from build123d import *

# Parameters (mm, degrees)
F0_R     = 12.942623
F1_DEPTH = 4.064
F4_DEPTH = 25.4
F5_DEPTH = 25.4


with BuildPart() as f1:
    # F0 (on Top) → F1 (new body)
    with BuildSketch(Plane.XY):
        Circle(F0_R)
    extrude(amount=F1_DEPTH)

    # F2 (on Top) → F4 (join)
    with BuildSketch(Plane.XY):
        Polygon((1.975973, 9.017531), (1.975973, 11.293087), (0.005284, 12.430865), (-1.965406, 11.293087), (-1.965406, 9.017531), (0.005284, 7.879752), align=None)
    extrude(amount=F4_DEPTH)

    # F3 (on face) → F5 (join)
    with BuildSketch(Plane.XY):
        Polygon((1.963999, -11.134515), (1.963999, -8.858958), (-0.006691, -7.72118), (-1.977381, -8.858958), (-1.977381, -11.134515), (-0.006691, -12.272293), align=None)
    extrude(amount=F5_DEPTH)


solid = f1.part
Input: part model. Units: mm. Frame: model coordinates. A direction names the side the tool comes from. Round coordinates to 2 decimals unless told otherwise and drop trailing zeros. Order: outer loops, then holes, each group sorted by start corner. A loop starts at its lowest first (then second) coordinate and runs counter-clockwise, first axis right, second up.
1. Cut plane D-D, the plane y = -9.5. Output: boundary loops of the cut face in (x, z), then the cut area to 3 significant figures.
The answers:
outline: (-8.79, 0) - (8.79, 0) - (8.79, 4.06) - (1.96, 4.06) - (1.96, 25.4) - (-1.98, 25.4) - (-1.98, 4.06) - (-8.79, 4.06) - close
area: 156 mm2
2. Cut plane B-B, the plane y = 0. Output: boundary loops of the cut face in (x, z), then the cut area to 3 significant figures.
The answers:
outline: (-12.94, 0) - (12.94, 0) - (12.94, 4.06) - (-12.94, 4.06) - close
area: 105 mm2
3. Material intervals for line 1 (Y direction, x = 0, z = 14.25); line 2 (Z direction, x = -6, y = 3); line 3 (X direction, y = -11.75, z = 2.25), sorted ascending.
The answers:
line 1: y = -12.27 to -7.73, 7.88 to 12.43
line 2: z = 0 to 4.06
line 3: x = -5.43 to 5.43
4. Mould query, pull axis Y, two halves, no side actions, for faces 6 (the face through (0.992, -8.298, 14.583)), 7 (the face through (1.004, 11.854, 14.583)), 8 (the face through (-1.977, -10, 15)). Classes: released by +Y, released by -Y, zero draft, split by the parting line, or undercut.
The answers:
face 6: undercut
face 7: released by +Y
face 8: zero draft
5. Cut plane A-A, the plane z = 16.75. Output: boundary loops of the cut face in (x, y).
The answers:
outline: (-1.98, -11.13) - (-0.01, -12.27) - (1.96, -11.13) - (1.96, -8.86) - (-0.01, -7.72) - (-1.98, -8.86) - close; (-1.97, 9.02) - (0.01, 7.88) - (1.98, 9.02) - (1.98, 11.29) - (0.01, 12.43) - (-1.97, 11.29) - close
6. Pin query (flat end, axial travel): P1, Ø1.8, axis at y = -10, z = 9.5, coming from the -X side; P2, Ø4, axis at y = 7.5, z = 13, coming from the +X side; P3, Ø5, axis at y = 5.5, z = 22, coming from the -X side. Return the tip coordinate at first contact, or that it passes through.
The answers:
P1: stops at x = -1.98
P2: stops at x = 1.98
P3: stops at x = -0.2
7. Cut plane C-C, the plane x = 6.75. Output: boundary loops of the cut face in (y, z), then the cut area to 3 significant figures.
The answers:
outline: (-11.04, 0) - (11.04, 0) - (11.04, 4.06) - (-11.04, 4.06) - close
area: 89.8 mm2
8. Set-up query: faces 1 (the face through (-0.978, -8.282, 14.583)), 2 (the face through (-1, -11.7, 14.6)), 3 (the face through (0.965, -11.711, 14.583)), 4 (the face through (0.977, 8.441, 14.583)), 5 (the face through (-0.97, 11.87, 14.58)). Return all of +Z, -Z, +X, -X, +Y, -Y with unobstructed straight access to the full face (end or side cutting, diameter ignored); none if empty.
The answers:
face 1: +Z, -X
face 2: +Z, -X, -Y
face 3: +Z, +X, -Y
face 4: +Z, +X
face 5: +Z, -X, +Y
